Input: dimensioned drawing with shaded views. Units: mm. Origin: part minimum x, y, z. Coordinates: 2 decimals unless noted, no trailing zeros. Write each loop counter-clockwise with the first axis right and the second up, starting at its lowest first coordinate (ties: lowest second). Pieces come first, ordered by that corner, then holes. Notation, with made-up numbers: (-15, 21) - (0, 21) arc R20 ccw to (0, 32) - close; hole circle Ø10 at (13.5, 38). An arc over 180 degrees is marked (long way). One line per question, with ' | ' between items.
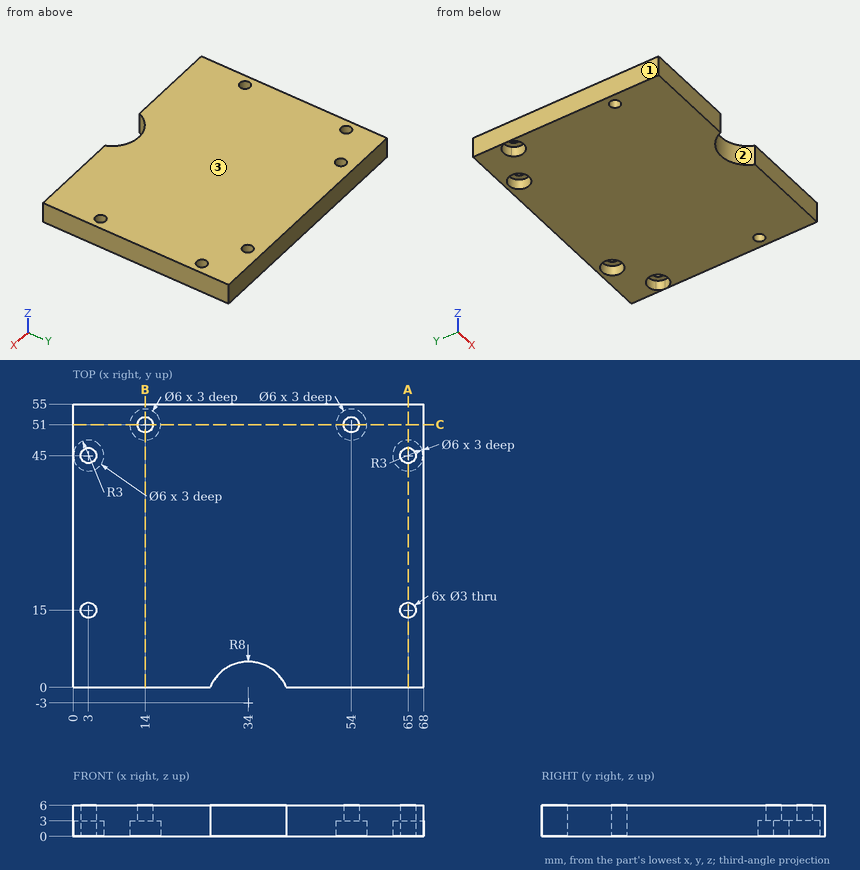
Item 1: Cut plane C-C on y = 51. Return loops of the section in (x, z).
Check sheet entries:
outline: (0, 0) - (11, 0) - (11, 3) - (12.5, 3) - (12.5, 6) - (0, 6) - close; (15.5, 3) - (17, 3) - (17, 0) - (51, 0) - (51, 3) - (52.5, 3) - (52.5, 6) - (15.5, 6) - close; (55.5, 3) - (57, 3) - (57, 0) - (68, 0) - (68, 6) - (55.5, 6) - close
Item 2: Mould query, pull axis X, two halves, no side actions, for the marked faces 1, 2 and 3. Classes: pulls with the +X half, pulls with the -X half, needs draft (parallel to the pull), parting line crosses it, or undercut.
Check sheet entries:
face 1: pulls with the -X half | face 2: undercut | face 3: needs draft
Item 3: Ray query, line 1 along X through (y, z) = (15, 4.2); line 2 along Y through (x, z) = (3, 3.85); line 3 along X through (y, z) = (51, 1.6). Return the intervals inside material, ascending. Write a range as [from, to].
Check sheet entries:
line 1: [0, 1.5], [4.5, 63.5], [66.5, 68] | line 2: [0, 13.5], [16.5, 43.5], [46.5, 55] | line 3: [0, 11], [17, 51], [57, 68]
Item 4: Cut plane B-B on x = 14. Return loops of the section in (y, z).
Check sheet entries:
outline: (0, 0) - (48, 0) - (48, 3) - (49.5, 3) - (49.5, 6) - (0, 6) - close; (52.5, 3) - (54, 3) - (54, 0) - (55, 0) - (55, 6) - (52.5, 6) - close
Item 5: Cut plane A-A on x = 65. Return loops of the section in (y, z).
Check sheet entries:
outline: (0, 0) - (13.5, 0) - (13.5, 6) - (0, 6) - close; (16.5, 0) - (42, 0) - (42, 3) - (43.5, 3) - (43.5, 6) - (16.5, 6) - close; (46.5, 3) - (48, 3) - (48, 0) - (55, 0) - (55, 6) - (46.5, 6) - close
Item 6: Pin query (flat end, axial travel): pin 1 Ø5 at (x, y) = (65, 45) entering from -Z. Return the tip coordinate at first contact, or that it passes through.
Check sheet entries:
pin 1: z = 3
